Design review of the part built by this model. Coordinates are the model's own, in mm. Give positions to 0.01 mm unless a question says otherwise; leave off trailing zeros. Order: outer loops, then holes, each group sorted by start corner. A loop starts at its lowest first (then second) coordinate and runs counter-clockwise, first axis right, second up. Notation, with made-up numbers: M 0.5,24.25 L 30.5,24.25 A10 cw 30.5,37.25 Z; hole C 30.25,88 d11. An arc over 180 degrees is marked long. Put each result on its own line as item: value. Start each with the question number.
from build123d import *

# Parameters (mm, degrees)
SKETCH_2_R         = 0.5
EXTRUDE_1_DEPTH    = 3.5
HOLE_WIZARD_M3_1_D = 2.5
HOLE_WIZARD_M4_1_D = 3.3
CHAMFER_1_SIZE     = 0.5


with BuildPart() as part:
    # 草图2 → 凸台-拉伸1 (new, symmetric)
    with BuildSketch(Plane.XY):
        with BuildLine():
            Line((3, 3), (3, -3))
            Line((3, -3), (-33.5, -3))
            ThreePointArc((-33.5, -3), (-36.5, 0), (-33.5, 3))
            Line((-33.5, 3), (3, 3))
        make_face()
        with Locations((-33.5, 0)):
            Circle(SKETCH_2_R, mode=Mode.SUBTRACT)
        with Locations((-24, 0)):
            Circle(SKETCH_2_R, mode=Mode.SUBTRACT)
        with Locations((-12, 0)):
            Circle(SKETCH_2_R, mode=Mode.SUBTRACT)
        Circle(SKETCH_2_R, mode=Mode.SUBTRACT)
    extrude(amount=EXTRUDE_1_DEPTH, both=True)

    # M3 螺纹孔1 (through all)
    with Locations(Plane.XY.offset(3.5)):
        with Locations((0, 0), (-12, 0), (-24, 0), (-33.5, 0)):
            Hole(HOLE_WIZARD_M3_1_D / 2)

    # M4 螺纹孔1 (through all)
    with Locations(Plane(origin=(0, 3, 0), x_dir=(1, 0, 0), z_dir=(0, 1, 0))):
        with Locations((-6, 0), (-18, 0)):
            Hole(HOLE_WIZARD_M4_1_D / 2)

    # 倒角1
    chamfer_1_edges = [part.edges().sort_by_distance(p)[0] for p in [
        (-15.25, -3, 3.5),
        (3, 0, 3.5),
        (-15.25, 3, 3.5),
        (3, 0, -3.5),
        (-15.25, -3, -3.5),
        (-36.5, 0, -3.5),
        (-15.25, 3, -3.5),
        (-36.5, 0, 3.5),
        (3, 3, 0),
        (3, -3, 0),
    ]]
    chamfer(chamfer_1_edges, length=CHAMFER_1_SIZE)


solid = part.part
1. Consider section C-C on z = 2.25. Give the boundary of the cut face in (x, y), then the cut area to 3 significant figures.
2. The part is to be moulded in two halves that separate along X. For faces 1 (the flat face through (-16, 0, 3.5)), 2 (the flat face through (3, 0, 0)), 3 (the cylindrical face through (-25.155, -0.479, -0.049)), say which applies: +X half, -X half, draft (parallel to the pull), parting line (faces both ways), or undercut.
3. Consider section B-B on x = 0. Give the boundary of the cut face in (y, z).
4. Consider section D-D on x = -18. Give the boundary of the cut face in (y, z).
5. Consider section A-A on z = 0. Give the boundary of the cut face in (x, y).
6. To check wall thickness, follow probe 1 along Y at (x, z) = (-24, 0.25); probe 2 along Z at (x, y) = (-18, -0.65); probe 3 along X at (y, z) = (1.65, -0.75). State the ranges of each line that lie inside material, in increasing order.
Returned:
1. outline: M -33.5,-3 L 2.5,-3 L 3,-2.5 L 3,2.5 L 2.5,3 L -33.5,3 A3 ccw Z; hole C -33.5,0 d2.5; hole C -24,0 d2.5; hole C -12,0 d2.5; hole C 0,0 d2.5
1. area: 213 mm2
2. face 1: draft
2. face 2: +X half
2. face 3: undercut
3. outline: M -3,-3 L -2.5,-3.5 L -1.25,-3.5 L -1.25,3.5 L -2.5,3.5 L -3,3 Z; M 1.25,-3.5 L 2.5,-3.5 L 3,-3 L 3,3 L 2.5,3.5 L 1.25,3.5 Z
4. outline: M -3,-3 L -2.5,-3.5 L 2.5,-3.5 L 3,-3 L 3,-1.65 L -3,-1.65 Z; M -3,1.65 L 3,1.65 L 3,3 L 2.5,3.5 L -2.5,3.5 L -3,3 Z
5. outline: M -33.5,-3 L -19.65,-3 L -19.65,3 L -33.5,3 A3 ccw Z; M -16.35,-3 L -7.65,-3 L -7.65,3 L -16.35,3 Z; M -4.35,-3 L 2.5,-3 L 3,-2.5 L 3,2.5 L 2.5,3 L -4.35,3 Z; hole C -33.5,0 d2.5; hole C -24,0 d2.5; hole C -12,0 d2.5; hole C 0,0 d2.5
6. probe 1: y = -3 to -1.25, 1.25 to 3
6. probe 2: z = -3.5 to -1.65, 1.65 to 3.5
6. probe 3: x = -36.01 to -19.47, -16.53 to -7.47, -4.53 to 3
